```python
from build123d import *

# Parameters (mm, degrees)
CROQUIS1_W                   = 35.4
CROQUIS1_H                   = 25.4
SALIENTE_EXTRUIR1_DEPTH      = 10
CROQUIS2_W                   = 7.4
CROQUIS2_H                   = 25.4
SALIENTE_EXTRUIR2_DEPTH      = 4
TALADRO_DE_MARGEN_PARA_M31_D = 3.4
CORTAR_EXTRUIR1_DEPTH        = 2
MATRIZL2_COUNT               = 2
MATRIZL2_PITCH               = 25.4
MATRIZL2_COUNT_DIR2          = 2
MATRIZL2_PITCH_DIR2          = 10.4


with BuildPart() as part:
    # Croquis1 → Saliente-Extruir1 (new body)
    with BuildSketch(Plane(origin=(0, 0, 0), x_dir=(1, 0, 0), z_dir=(0, 1, 0))):
        Rectangle(CROQUIS1_W, CROQUIS1_H)
    extrude(amount=SALIENTE_EXTRUIR1_DEPTH)

    # Croquis2 → Saliente-Extruir2 (add)
    with BuildSketch(Plane(origin=(0, 10, 0), x_dir=(1, 0, 0), z_dir=(0, 1, 0))):
        with Locations((-14, 0)):
            Rectangle(CROQUIS2_W, CROQUIS2_H)
    saliente_extruir2 = extrude(amount=SALIENTE_EXTRUIR2_DEPTH)

    # Simetría1: Saliente-Extruir2 across plane
    add(saliente_extruir2.mirror(Plane(origin=(0, 0, 0), x_dir=(0, 0, 1), z_dir=(1, 0, 0))))

    # Taladro de margen para M31 (through all)
    with Locations(Plane(origin=(0, 14, 0), x_dir=(1, 0, 0), z_dir=(0, 1, 0))):
        with Locations((-12.7, 5.2), (12.7, -5.2), (12.7, 5.2), (-12.7, -5.2)):
            Hole(TALADRO_DE_MARGEN_PARA_M31_D / 2)

    # Croquis6 → Cortar-Extruir1 (cut)
    with BuildSketch(Plane.XZ):
        Polygon((-9.7, 6.932050808), (-12.7, 8.664101615), (-15.7, 6.932050808), (-15.7, 3.467949192), (-12.7, 1.735898385), (-9.7, 3.467949192), align=None)
    cortar_extruir1 = extrude(amount=-CORTAR_EXTRUIR1_DEPTH, mode=Mode.SUBTRACT)

    # MatrizL2: Cortar-Extruir1 2 × 2
    with Locations(*[(i * MATRIZL2_PITCH, 0, -j * MATRIZL2_PITCH_DIR2) for i in range(MATRIZL2_COUNT) for j in range(MATRIZL2_COUNT_DIR2) if (i, j) != (0, 0)]):
        add(cortar_extruir1, mode=Mode.SUBTRACT)


solid = part.part
```
Work out the finished part from the listing and answer in its coordinate system (mm). A direction names the side the tool comes from. Give positions to 0.01 mm unless a question says otherwise; leave off trailing zeros. Order: outer loops, then holes, each group sorted by start corner. A loop starts at its lowest first (then second) coordinate and runs counter-clockwise, first axis right, second up.
1. Straight lines are drawn through the part: L1, parallel to Z at x = 12.7, y = 9.5; L2, parallel to X at y = 8, z = -5.2; L3, parallel to X at y = 11.75, z = -5.2. For each, find the intervals that lie inside material, in ascending order.
Result sheet:
L1: z = -12.7 to -6.9, -3.5 to 3.5, 6.9 to 12.7
L2: x = -17.7 to -14.4, -11 to 11, 14.4 to 17.7
L3: x = -17.7 to -14.4, -11 to -10.3, 10.3 to 11, 14.4 to 17.7
2. Section B-B, the plane y = 2.5 is taken. Determine the outline of the cut face in (x, z), and give its area (3 significant figures).
Result sheet:
outline: (-17.7, -12.7) - (17.7, -12.7) - (17.7, 12.7) - (-17.7, 12.7) - close; hole circle Ø3.4 at (-12.7, -5.2); hole circle Ø3.4 at (-12.7, 5.2); hole circle Ø3.4 at (12.7, -5.2); hole circle Ø3.4 at (12.7, 5.2)
area: 863 mm2
3. Each of these flat-tipped pins is pushed along its axis until it touches: P1, Ø4, axis at x = -12.7, z = 5.2, coming from the -Y side; P2, Ø3, axis at x = 12.7, z = -5.2, coming from the +Y side; P3, Ø5, axis at x = 5.5, z = 8, coming from the +Y side. Where does it stop, or does it pass through?
Result sheet:
P1: stops at y = 2
P2: passes through
P3: stops at y = 10
4. For faces 3 (the cylindrical face through (12.921, 7.916, -6.886)), 4 (the flat face through (10.3, 12, 0)), 5 (the flat face through (-15.7, 1, 5)), determine the directions among +Z, -Z, +X, -X, +Y, -Y from which every point of the face is accessible in a straight line to the end or side of a thin tool.
Result sheet:
face 3: +Y, -Y
face 4: +Z, -Z, +Y
face 5: -Y
5. Section D-D, the plane z = 7.75 is taken. Determine the outline of the cut face in (x, y).
Result sheet:
outline: (-17.7, 0) - (-14.28, 0) - (-14.28, 2) - (-11.12, 2) - (-11.12, 0) - (11.12, 0) - (11.12, 2) - (14.28, 2) - (14.28, 0) - (17.7, 0) - (17.7, 14) - (10.3, 14) - (10.3, 10) - (-10.3, 10) - (-10.3, 14) - (-17.7, 14) - close
6. Section A-A, the plane z = -5.2 is taken. Determine the outline of the cut face in (x, y).
Result sheet:
outline: (-17.7, 0) - (-15.7, 0) - (-15.7, 2) - (-14.4, 2) - (-14.4, 14) - (-17.7, 14) - close; (-11, 2) - (-9.7, 2) - (-9.7, 0) - (9.7, 0) - (9.7, 2) - (11, 2) - (11, 14) - (10.3, 14) - (10.3, 10) - (-10.3, 10) - (-10.3, 14) - (-11, 14) - close; (14.4, 2) - (15.7, 2) - (15.7, 0) - (17.7, 0) - (17.7, 14) - (14.4, 14) - close
7. Section C-C, the plane x = 3 is taken. Determine the outline of the cut face in (y, z).
Result sheet:
outline: (0, -12.7) - (10, -12.7) - (10, 12.7) - (0, 12.7) - close
8. The mould has two halves that part along X. Classify faces 1 (the flat face through (-9.7, 1, 5)), 2 (the flat face through (0, 5, -12.7)): released by +X, released by -X, zero draft, split by the parting line, or undercut.
Result sheet:
face 1: undercut
face 2: zero draft
